from build123d import *

# Parameters (mm, degrees)
SKETCH_1_W      = 55
SKETCH_1_H      = 55
EXTRUDE_1_DEPTH = 55
SKETCH_2_R      = 2.5
EXTRUDE_2_DEPTH = 10
SKETCH_3_R      = 2.5
EXTRUDE_3_DEPTH = 10
FILLET_1_R      = 20


with BuildPart() as part:
    # Эскиз1 → Бобышка-Вытянуть1 (new body)
    with BuildSketch(Plane.XY):
        with Locations((-11.523913591, 5.040193617)):
            Rectangle(SKETCH_1_W, SKETCH_1_H)
    extrude(amount=EXTRUDE_1_DEPTH)

    # Эскиз2 → Бобышка-Вытянуть2 (add)
    with BuildSketch(Plane(origin=(15.976086409, 0, 0), x_dir=(0, 0, -1), z_dir=(1, 0, 0))):
        with Locations((-7.523581631, 5.040193617)):
            Circle(SKETCH_2_R)
    extrude(amount=EXTRUDE_2_DEPTH)

    # Эскиз3 → Бобышка-Вытянуть3 (add)
    with BuildSketch(Plane.XY.offset(55)):
        with Locations((-11.523913591, 5.040193617)):
            Circle(SKETCH_3_R)
    extrude(amount=EXTRUDE_3_DEPTH)

    # Скругление1
    fillet_1_edges = [part.edges().sort_by_distance(p)[0] for p in [
        (-11.523913591, 32.540193617, 55),
        (-11.523913591, 32.540193617, 0),
        (-11.523913591, -22.459806383, 0),
        (-11.523913591, -22.459806383, 55),
    ]]
    fillet(fillet_1_edges, radius=FILLET_1_R)


solid = part.part
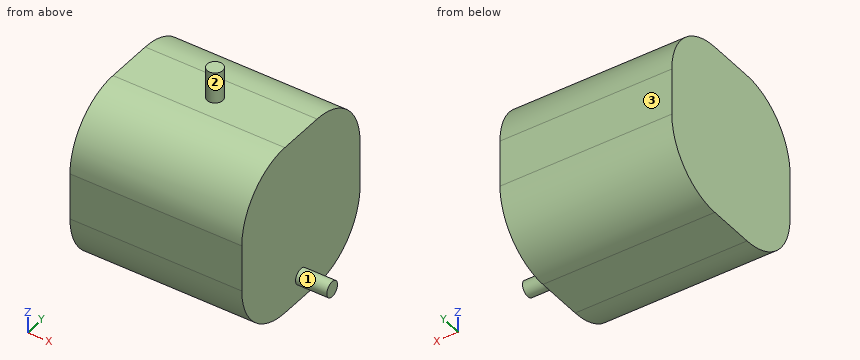
Read the model definition and answer for the solid it produces. Units are mm, in the model's axes. Face numbers are marked on the shaded views. A direction names the side the tool comes from. Give positions to 0.01 mm unless a question says otherwise; leave off trailing zeros. Loops run counter-clockwise (first coordinate to the right, second up) from the corner with the lowest first, then second, coordinate; pieces in that order, holes last. Notation, with made-up numbers: (-33, 3.5) -> (23, 3.5) arc R15 ccw to (23, 9.5) -> close; hole circle Ø1 at (57, 46). An arc over 180 degrees is marked (long way). Use a Markdown table: item, result.
Q1. Section B-B, the plane z = 30 is taken. Determine the outline of the cut face in (x, y).
Solved:
| item | result |
|---|---|
| outline | (-39.02, -22.46) -> (15.98, -22.46) -> (15.98, 32.54) -> (-39.02, 32.54) -> close |
Q2. A tool of negligible diameter and unlimited length cuts with its end or side. For the marked faces 1, 2 and 3, from which of +Z, -Z, +X, -X, +Y, -Y can it reach the whole face along a straight path? Write none if from no direction.
Solved:
| item | result |
|---|---|
| face 1 | +X |
| face 2 | +Z |
| face 3 | +Z, -Z, +X, -X, +Y |
Q3. Section C-C, the plane y = 9.5 is taken. Determine the outline of the cut face in (x, z), then the cut area to 4 significant figures.
Solved:
| item | result |
|---|---|
| outline | (-39.02, 0) -> (15.98, 0) -> (15.98, 55) -> (-39.02, 55) -> close |
| area | 3,025 mm^2 |
Q4. Section D-D, the plane x = -10.5 is taken. Determine the outline of the cut face in (y, z).
Solved:
| item | result |
|---|---|
| outline | (-22.46, 20) arc R20 ccw to (-2.46, 0) -> (12.54, 0) arc R20 ccw to (32.54, 20) -> (32.54, 35) arc R20 ccw to (12.54, 55) -> (7.32, 55) -> (7.32, 65) -> (2.76, 65) -> (2.76, 55) -> (-2.46, 55) arc R20 ccw to (-22.46, 35) -> close |
Q5. Section A-A, the plane x = 5.5 is taken. Determine the outline of the cut face in (y, z).
Solved:
| item | result |
|---|---|
| outline | (-22.46, 20) arc R20 ccw to (-2.46, 0) -> (12.54, 0) arc R20 ccw to (32.54, 20) -> (32.54, 35) arc R20 ccw to (12.54, 55) -> (-2.46, 55) arc R20 ccw to (-22.46, 35) -> close |
Q6. Each of these flat-tipped pins is pushed along its axis until it touches: pin 1 (3 mm diameter, centred on x = -18.5, z = 9, fed in from +Y); pin 2 (3 mm diameter, centred on x = -30, y = -9.5, fed in from -Z); pin 3 (12 mm diameter, centred on x = -24.5, y = 4.5, fed in from +Z). Where does it stop, or does it pass through?
Solved:
| item | result |
|---|---|
| pin 1 | stops at y = 30.14 |
| pin 2 | stops at z = 0.78 |
| pin 3 | stops at z = 55 |
Q7. Find the intervals of material crossed by line 1 along X through (y, z) = (15, 25); line 2 along Z through (x, y) = (-0.5, 3); line 3 along Z through (x, y) = (-19, -17), in increasing order.
Solved:
| item | result |
|---|---|
| line 1 | x = -39.02 to 15.98 |
| line 2 | z = 0 to 55 |
| line 3 | z = 6.27 to 48.73 |
